Answer from the drawing. Dimensions are ordinates in mm from the lowest x, y and z of the part. A direction names the side the tool comes from. Give positions to 0.01 mm unless a question says otherwise; leave off trailing zeros. Loops run counter-clockwise (first coordinate to the right, second up) from the corner with the lowest first, then second, coordinate; pieces in that order, holes last.
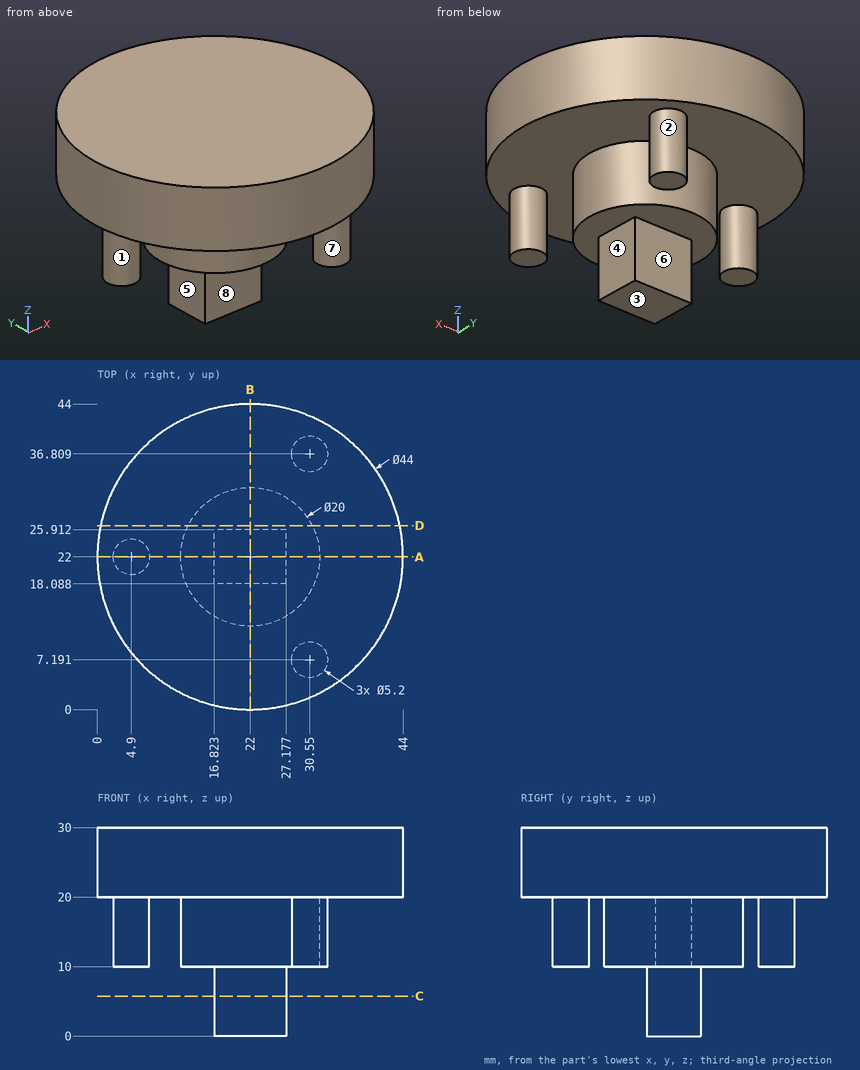
Item 1: Find section B-B, the plane x = 22. Write down the section's boundary in (y, z), plus the area to 3 significant figures.
Item 2: Flat-ended cylindrical pins translate along their axes: pin 1 Ø2 at (x, y) = (13.5, 36.5) entering from -Z; pin 2 Ø8 at (x, z) = (21, 5) entering from +Y; pin 3 Ø1.6 at (x, y) = (30, 8.5) entering from -Z. Find the tip coordinate at first contact, or state that the pin passes through.
Item 3: Determine the mould class of the marked faces 1, 2, 3 and 4 for opening direction X: released by +X, released by -X, zero draft, split by the parting line, or undercut.
Item 4: Find section A-A, the plane y = 22. Write down the section's boundary in (x, z).
Item 5: Find section D-D, the plane y = 26.5. Write down the section's boundary in (x, z) (1 decimal).
Item 6: Find section C-C, the plane z = 5.75. Write down the section's boundary in (x, y).
Item 7: Consider line 1 (Z direction, x = 32.5, y = 23); line 2 (Y direction, x = 19, z = 9.5); line 3 (Z direction, x = 29, y = 23.5). Determine where each line is inside the solid, lowest interval first.
Item 8: For the marked faces 5, 6, 7 and 8, determine the directions among +Z, -Z, +X, -X, +Y, -Y from which every point of the face is accessible in a straight line to the end or side of a thin tool.
Ans:
1. outline: (0, 20) - (12, 20) - (12, 10) - (18.09, 10) - (18.09, 0) - (25.91, 0) - (25.91, 10) - (32, 10) - (32, 20) - (44, 20) - (44, 30) - (0, 30) - close
1. area: 718 mm2
2. pin 1: stops at z = 20
2. pin 2: stops at y = 25.91
2. pin 3: stops at z = 10
3. face 1: undercut
3. face 2: split by the parting line
3. face 3: zero draft
3. face 4: released by +X
4. outline: (0, 20) - (2.3, 20) - (2.3, 10) - (7.5, 10) - (7.5, 20) - (12, 20) - (12, 10) - (16.82, 10) - (16.82, 0) - (27.18, 0) - (27.18, 10) - (32, 10) - (32, 20) - (44, 20) - (44, 30) - (0, 30) - close
5. outline: (0.5, 20) - (13.1, 20) - (13.1, 10) - (30.9, 10) - (30.9, 20) - (43.5, 20) - (43.5, 30) - (0.5, 30) - close
6. outline: (16.82, 18.09) - (27.18, 18.09) - (27.18, 25.91) - (16.82, 25.91) - close
7. line 1: z = 20 to 30
7. line 2: y = 18.09 to 25.91
7. line 3: z = 10 to 30
8. face 5: -Z, -X, +Y, -Y
8. face 6: -Z, +X, -X, +Y
8. face 7: -Z
8. face 8: -Z, +X, -X, -Y
